CAD build for the part. Positions are in the model's coordinates, mm. A direction names the side the tool comes from. Round coordinates to 2 decimals unless told otherwise and drop trailing zeros. Put each result on its own line as item: value.
```python
from build123d import *

# Parameters (mm, degrees)
F0_W        = 18.9
F0_H        = 9.6
F0_W_2      = 15.9
F0_H_2      = 3.1
F1_DEPTH    = 1.2
F2_SIZE     = 1.19999
F3_T1_DEPTH = 4.9651949945
F3_T3_DEPTH = 4.9651949945
F3_T5_DEPTH = 4.9651949945
F3_T7_DEPTH = 4.9651949945


# Not quite as in the source:
# - a fillet or chamfer that OpenCascade refuses, or shapes differently, is made with other operations: its cross-section is extruded or revolved along the edge and cut away or added
# - a fillet or chamfer is up to 0.001 mm smaller than in the source, because OpenCascade refuses the exact size


with BuildPart() as f1:
    # F0 (on Top) → F1 (new body)
    with BuildSketch(Plane.XY):
        Rectangle(F0_W, F0_H)
        with Locations((0, -1.75)):
            Rectangle(F0_W_2, F0_H_2, mode=Mode.SUBTRACT)
        with Locations((0, 1.75)):
            Rectangle(F0_W_2, F0_H_2, mode=Mode.SUBTRACT)
    extrude(amount=F1_DEPTH)

    # F2 (size 1.2 in the source; OpenCascade refuses exactly that, so slightly less here)
    f2_edges = [f1.edges().sort_by_distance(p)[0] for p in [
        (0, -4.8, 1.2),
        (-9.45, 0, 1.2),
        (9.45, 0, 1.2),
        (0, 4.8, 1.2),
    ]]
    chamfer(f2_edges, length=F2_SIZE)

    # F3: fillet of radius 1 on 4 edges, made by hand

    # F3_s2 → F3_t1 (cut)
    with BuildSketch(Plane(origin=(-5.58333, -5.58333, -5.58333), x_dir=(-0.7071067812, 0.7071067812, 0), z_dir=(0.5773502692, 0.5773502692, 0.5773502692))):
        with BuildLine():
            ThreePointArc((3.7880465325, 5.5288711695), (3.2880465325, 5.6628457657), (2.7880465325, 5.5288711695))
            Line((2.7880465325, 5.5288711695), (3.2880465325, 5.8175463041))
            Line((3.2880465325, 5.8175463041), (3.7880465325, 5.5288711695))
        make_face()
    extrude(amount=F3_T1_DEPTH, mode=Mode.SUBTRACT)

    # F3_s4 → F3_t3 (cut)
    with BuildSketch(Plane(origin=(5.58333, -5.58333, -5.58333), x_dir=(-0.7071067812, -0.7071067812, 0), z_dir=(-0.5773502692, 0.5773502692, 0.5773502692))):
        with BuildLine():
            ThreePointArc((-3.7880465325, 5.5288711695), (-3.2880465325, 5.6628457657), (-2.7880465325, 5.5288711695))
            Line((-2.7880465325, 5.5288711695), (-3.2880465325, 5.8175463041))
            Line((-3.2880465325, 5.8175463041), (-3.7880465325, 5.5288711695))
        make_face()
    extrude(amount=F3_T3_DEPTH, mode=Mode.SUBTRACT)

    # F3_s6 → F3_t5 (cut)
    with BuildSketch(Plane(origin=(5.58333, 5.58333, -5.58333), x_dir=(0.7071067812, -0.7071067812, 0), z_dir=(-0.5773502692, -0.5773502692, 0.5773502692))):
        with BuildLine():
            ThreePointArc((2.7880465325, 5.5288711695), (3.2880465325, 5.6628457657), (3.7880465325, 5.5288711695))
            Line((3.7880465325, 5.5288711695), (3.2880465325, 5.8175463041))
            Line((3.2880465325, 5.8175463041), (2.7880465325, 5.5288711695))
        make_face()
    extrude(amount=F3_T5_DEPTH, mode=Mode.SUBTRACT)

    # F3_s8 → F3_t7 (cut)
    with BuildSketch(Plane(origin=(-5.58333, 5.58333, -5.58333), x_dir=(0.7071067812, 0.7071067812, 0), z_dir=(0.5773502692, -0.5773502692, 0.5773502692))):
        with BuildLine():
            ThreePointArc((-2.7880465325, 5.5288711695), (-3.2880465325, 5.6628457657), (-3.7880465325, 5.5288711695))
            Line((-3.7880465325, 5.5288711695), (-3.2880465325, 5.8175463041))
            Line((-3.2880465325, 5.8175463041), (-2.7880465325, 5.5288711695))
        make_face()
    extrude(amount=F3_T7_DEPTH, mode=Mode.SUBTRACT)


solid = f1.part
```
Item 1: Pin check, flat tips, straight feed: P1, Ø0.6, axis at y = 1.5, z = 0.5, coming from the -X side; P2, Ø0.6, axis at y = -2.5, z = 1, coming from the +X side; P3, Ø0.6, axis at y = -1, z = 1, coming from the -X side. Stop position of each tip, or through.
Answers below:
P1: x = -9.25
P2: x = 8.75
P3: x = -8.75
Item 2: Probe line 1 along Y through (x, z) = (-1.5, 0.7); line 2 along Y through (x, z) = (-2.5, 0.5); line 3 along X through (y, z) = (3.25, 0.4). List the from-to ranges inside material, lowest first. Write a range as [from, to].
Answers below:
line 1: [-4.1, -3.3], [-0.2, 0.2], [3.3, 4.1]
line 2: [-4.3, -3.3], [-0.2, 0.2], [3.3, 4.3]
line 3: [-9.05, -7.95], [7.95, 9.05]
Item 3: Mould opens along Y. For faces 3 (the flat face through (0, 3.3, 1)), 4 (the flat face through (-8.84, -0.06, 0.61)), 5 (the flat face through (-0.1, 4.2, 0.6)) say: pulls with the +Y half, pulls with the -Y half, needs draft (parallel to the pull), parting line crosses it, or undercut.
Answers below:
face 3: undercut
face 4: needs draft
face 5: pulls with the +Y half
Item 4: Band-saw the part on A-A on x = -3. State how many separate pieces and enclosed holes the cut face has, and give its area (3 significant figures).
Answers below:
separate pieces: 3
enclosed holes: 0
area: 2.64 mm²
Item 5: Tool access for faces 1 (the flat face through (0, -0.2, 1)), 2 (the cylindrical face through (-8.632, -3.971, 0.634)): list every direction of +Z, -Z, +X, -X, +Y, -Y with a clear straight run to the whole face (end or side of a thin tool).
Answers below:
face 1: +Z, -Z
face 2: +Z, -X, -Y
